Work out the finished part from the listing and answer in its coordinate system (mm). Coordinates: 2 decimals unless noted, no trailing zeros. Loops run counter-clockwise (first coordinate to the right, second up) from the corner with the lowest first, then second, coordinate; pieces in that order, holes last. Notation, with made-up numbers: (-24, 27) - (-3, 27) arc R13 cw to (-3, 52) - close; hole circle Ø2 at (-14.5, -33.5). An arc over 180 degrees is marked (long way). Write each question's results on one line, items separated by ' | '. Start each with the question number.
1. Determine the mould class of faces 1 (the cylindrical face through (19.515, -7.731, 2.958)), 2 (the flat face through (20, 0, 0)), 3 (the cylindrical face through (22.946, 21.157, 1.203)) for opening direction X: released by +X, released by -X, zero draft, split by the parting line, or undercut.
2. Each of these flat-tipped pins is pushed along its axis until it touches: P1, Ø1, axis at y = 8, z = 4, coming from the +X side; P2, Ø2, axis at y = -18.5, z = 3.5, coming from the -X side; P3, Ø2, axis at y = -18.5, z = 3, coming from the -X side. Where does it stop, or does it pass through?
3. A cutting plane is placed at C-C on z = 1.25. State how many separate pieces and enclosed holes the cut face has, then the cut area to 3 significant figures.
4. A cutting plane is placed at A-A on x = 0. Determine the outline of the cut face in (y, z), then the cut area to 3 significant figures.
5. Find the intervals of material crossed by line 1 along X through (y, z) = (6, 3.5); line 2 along X through (y, z) = (3, 4.75); line 3 along X through (y, z) = (8.5, 2.75), in increasing order. Write a range as [from, to].
6. A cutting plane is placed at B-B on y = 0. Determine the outline of the cut face in (x, z), then the cut area to 3 significant figures.
from build123d import *

# Parameters (mm, degrees)
SKETCH1_R           = 2.15
SKETCH1_R_2         = 1.6
SKETCH1_R_3         = 2.1
SKETCH1_R_4         = 2.65
SKETCH1_R_5         = 18.5625
SKETCH1_R_6         = 15.0625
BOSS_EXTRUDE1_DEPTH = 6
FILLET1_R           = 4


with BuildPart() as part:
    # Sketch1 → Boss-Extrude1 (new body)
    with BuildSketch(Plane.XY):
        with BuildLine():
            Line((3.125, -24.803918541), (42.5, -19.843134833))
            ThreePointArc((42.5, -19.843134833), (60, 0), (42.5, 19.843134833))
            Line((42.5, 19.843134833), (3.125, 24.803918541))
            ThreePointArc((3.125, 24.803918541), (-25, 0), (3.125, -24.803918541))
        make_face()
        with Locations((21.663293527, -7.825180806)):
            Circle(SKETCH1_R, mode=Mode.SUBTRACT)
        with Locations((22.126671777, 7.712150618)):
            Circle(SKETCH1_R_2, mode=Mode.SUBTRACT)
        with Locations((24.253343554, 15.424301236)):
            Circle(SKETCH1_R_3, mode=Mode.SUBTRACT)
        with Locations((23.326587053, -15.650361612)):
            Circle(SKETCH1_R_4, mode=Mode.SUBTRACT)
        Circle(SKETCH1_R_5, mode=Mode.SUBTRACT)
        with Locations((40, 0)):
            Circle(SKETCH1_R_6, mode=Mode.SUBTRACT)
    extrude(amount=BOSS_EXTRUDE1_DEPTH)

    # Fillet1
    # the kernel refuses this fillet: 4 mm, written as the material it takes off along each edge
    with BuildSketch(Plane(origin=(0, 0, 0), x_dir=(0.12499999999999982, 0.9921567416492215, 0), z_dir=(0.9921567416492215, -0.12499999999999982, 0))) as fillet1_piece_1:
        with BuildLine():
            CenterArc((25 - FILLET1_R, FILLET1_R), FILLET1_R, 270, 90)
            Line((25 - FILLET1_R, 0), (25, 0))
            Line((25, 0), (25, FILLET1_R))
        make_face()
    revolve(axis=Axis((0, 0, 0), (0, 0, 1)), revolution_arc=194.361511563, mode=Mode.SUBTRACT)
    with BuildSketch(Plane(origin=(42.5, 19.843134833, 0), x_dir=(0, 0, 1), z_dir=(-0.9921567416492215, 0.12500000000000022, 0)), Plane(origin=(3.125, -24.803918541, 0), x_dir=(0, 0, 1), z_dir=(0.9921567416492215, 0.12500000000000014, 0))) as fillet1_piece_2:
        with BuildLine():
            CenterArc((FILLET1_R, -FILLET1_R), FILLET1_R, 90, 90)
            Line((0, -FILLET1_R), (0, 0))
            Line((0, 0), (FILLET1_R, 0))
        make_face()
    extrude(amount=39.686269666, mode=Mode.SUBTRACT)
    with BuildSketch(Plane(origin=(40, 0, 0), x_dir=(0.12499999999999938, -0.9921567416492216, 0), z_dir=(-0.9921567416492216, -0.12499999999999938, 0))) as fillet1_piece_3:
        with BuildLine():
            CenterArc((20 - FILLET1_R, FILLET1_R), FILLET1_R, 270, 90)
            Line((20 - FILLET1_R, 0), (20, 0))
            Line((20, 0), (20, FILLET1_R))
        make_face()
    revolve(axis=Axis((40, 0, 0), (0, 0, 1)), revolution_arc=165.638488437, mode=Mode.SUBTRACT)


solid = part.part
Values:
1) face 1: undercut | face 2: zero draft | face 3: released by +X
2) P1: x = 58.54 | P2: x = -17.82 | P3: x = -17.72
3) separate pieces: 1 | enclosed holes: 6 | area: 1,330 mm^2
4) outline: (-25, 4) arc R4 ccw to (-21, 0) - (-18.56, 0) - (-18.56, 6) - (-25, 6) - close; (18.56, 0) - (21, 0) arc R4 ccw to (25, 4) - (25, 6) - (18.56, 6) - close | area: 70.4 mm^2
5) line 1: [-24.24, -17.57], [17.57, 26.18], [53.82, 59.05] | line 2: [-24.82, -18.32], [18.32, 25.24], [54.76, 59.77] | line 3: [-23.3, -16.5], [16.5, 20.73], [23.52, 27.57], [52.43, 57.88]
6) outline: (-25, 4) arc R4 ccw to (-21, 0) - (-18.56, 0) - (-18.56, 6) - (-25, 6) - close; (18.56, 0) - (24.94, 0) - (24.94, 6) - (18.56, 6) - close; (55.06, 0) - (56, 0) arc R4 ccw to (60, 4) - (60, 6) - (55.06, 6) - close | area: 99.6 mm^2
